from build123d import *

# Parameters (mm, degrees)
BASE_FLANGE1_START                       = -12.7
BASE_FLANGE1_OUTLINE_W                   = 1219.2
BASE_FLANGE1_OUTLINE_H                   = 685.8
BASE_FLANGE1_DEPTH                       = 12.7
CBORE_FOR_M8_SHCS1_D                     = 9
CBORE_FOR_M8_SHCS1_CBORE_D               = 17
CBORE_FOR_M8_SHCS1_CBORE_DEPTH           = 8
CBORE_FOR_M6_SHCS1_D                     = 6.6
CBORE_FOR_M6_SHCS1_CBORE_D               = 11
CBORE_FOR_M6_SHCS1_CBORE_DEPTH           = 6
CBORE_FOR_M10_HEX_HEAD_BOLT1_D           = 11
CBORE_FOR_M10_HEX_HEAD_BOLT1_CBORE_D     = 21.48
CBORE_FOR_M10_HEX_HEAD_BOLT1_CBORE_DEPTH = 6.85


# Read off the part's stored shape, not the designer's step: Base-Flange1
with BuildPart() as part:
    # Base-Flange1 outline → Base-Flange1 (new body)
    with BuildSketch(Plane(origin=(0, 0, 0), x_dir=(1, 0, 0), z_dir=(0, 1, 0)).offset(BASE_FLANGE1_START)):
        Rectangle(BASE_FLANGE1_OUTLINE_W, BASE_FLANGE1_OUTLINE_H)
    extrude(amount=BASE_FLANGE1_DEPTH)

    # CBORE for M8 SHCS1 (through all)
    with Locations(Plane(origin=(0, -12.7, 0), x_dir=(-1, 0, 0), z_dir=(0, -1, 0))):
        with Locations((-499.6, -92.9), (0, 312.9), (-250, 312.9), (-500, 312.9), (500, 312.9), (250, 312.9), (500, -312.9), (250, -312.9), (0, -312.9), (-250, -312.9), (-500, -312.9), (-579.6, 125), (-579.6, -125), (579.6, -125), (579.6, 125), (-459.6, 13.7), (-559.6, 13.7), (-539.6, -132.9), (574.6, 13.7), (494.6, 13.7), (100.4, 282.9), (20.4, 282.9), (60.4, 322.9), (-497.6, -26.3), (-497.6, 53.7), (-369.556226637, -134.809538036), (-499.6, -172.9)):
            CounterBoreHole(CBORE_FOR_M8_SHCS1_D / 2, CBORE_FOR_M8_SHCS1_CBORE_D / 2, CBORE_FOR_M8_SHCS1_CBORE_DEPTH)

    # CBORE for M6 SHCS1 (through all)
    with Locations(Plane(origin=(0, -12.7, 0), x_dir=(-1, 0, 0), z_dir=(0, -1, 0))):
        with Locations((184.85, 255.6), (184.85, 230.2), (162.625, 230.2), (162.625, 255.6), (162.625, -237.5), (162.625, -262.9), (141.573996145, -237.577193976), (140.4, -237.5), (140.4, -262.9), (-146.9, -117.9), (-172.3, -117.9), (-172.3, -95.675), (-146.9, -95.675), (-146.9, 120.675), (-172.3, 120.675), (-172.3, 142.9), (-146.9, 142.9)):
            CounterBoreHole(CBORE_FOR_M6_SHCS1_D / 2, CBORE_FOR_M6_SHCS1_CBORE_D / 2, CBORE_FOR_M6_SHCS1_CBORE_DEPTH)

    # CBORE for M10 Hex Head Bolt1 (through all)
    with Locations(Plane(origin=(0, -12.7, 0), x_dir=(-1, 0, 0), z_dir=(0, -1, 0))):
        with Locations((-309.6, 13.7), (-309.6, -132.9)):
            CounterBoreHole(CBORE_FOR_M10_HEX_HEAD_BOLT1_D / 2, CBORE_FOR_M10_HEX_HEAD_BOLT1_CBORE_D / 2, CBORE_FOR_M10_HEX_HEAD_BOLT1_CBORE_DEPTH)


solid = part.part
Model file for the job. Use its own axes, mm. A direction names the side the tool comes from. Coordinates: 2 decimals unless noted, no trailing zeros. Return JSON: item names as keys, results as strings.
1. Flat gauge pins, fed straight in: pin 1 (13.5 mm diameter, centred on x = -500, z = 312.9, fed in from -Y); pin 2 (8.5 mm diameter, centred on x = 146.9, z = 95.675, fed in from -Y). Where does each tip first touch, or does it go through?
Ans:
{"pin 1": "y = -4.7", "pin 2": "y = -6.7"}
2. Drill centre lines: probe 1 along X at (y, z) = (-10.45, -230.2) (3 decimals); probe 2 along X at (y, z) = (-3.25, 238); probe 3 along Z at (x, y) = (0, -3.6). Where is each one in solid material? Low to high.
Ans:
{"probe 1": "-609.6 to -190.35, -179.35 to -168.125, -157.125 to 609.6", "probe 2": "-609.6 to -165.89, -159.36 to -144.85, -137.14 to 609.6", "probe 3": "-342.9 to -317.4, -308.4 to 308.4, 317.4 to 342.9"}
3. Pull direction Z, two halves, no side cores. Call faces 3 (the face through (299.356, -9.323, -16.926)), 4 (the face through (-9, 0, -5)): +Z half, -Z half, draft (parallel to the pull), parting line (faces both ways), or undercut.
Ans:
{"face 3": "undercut", "face 4": "draft"}
4. Tool access for faces 1 (the face through (-9, -12.7, -5)), 2 (the face through (315, -5.85, 130)): list every direction of +Z, -Z, +X, -X, +Y, -Y with a clear straight run to the whole face (end or side of a thin tool).
Ans:
{"face 1": "+Z, -Z, +X, -X, -Y", "face 2": "-Y"}
